Source: three-view drawing plus pictorial views. Frame: mm from the lowest corner of the part. Give positions to 0.01 mm unless a question says otherwise; leave off trailing zeros. Write each loop counter-clockwise with the first axis right and the second up, starting at its lowest first coordinate (ties: lowest second). Pieces come first, ordered by that corner, then holes. Notation, with made-up numbers: M -33.5,-4.75 L -21.5,-4.75 A25 ccw -21.5,9.25 Z; hole C 46.5,76 d5. An arc over 180 degrees is marked long. Return JSON: item names as keys, results as strings.
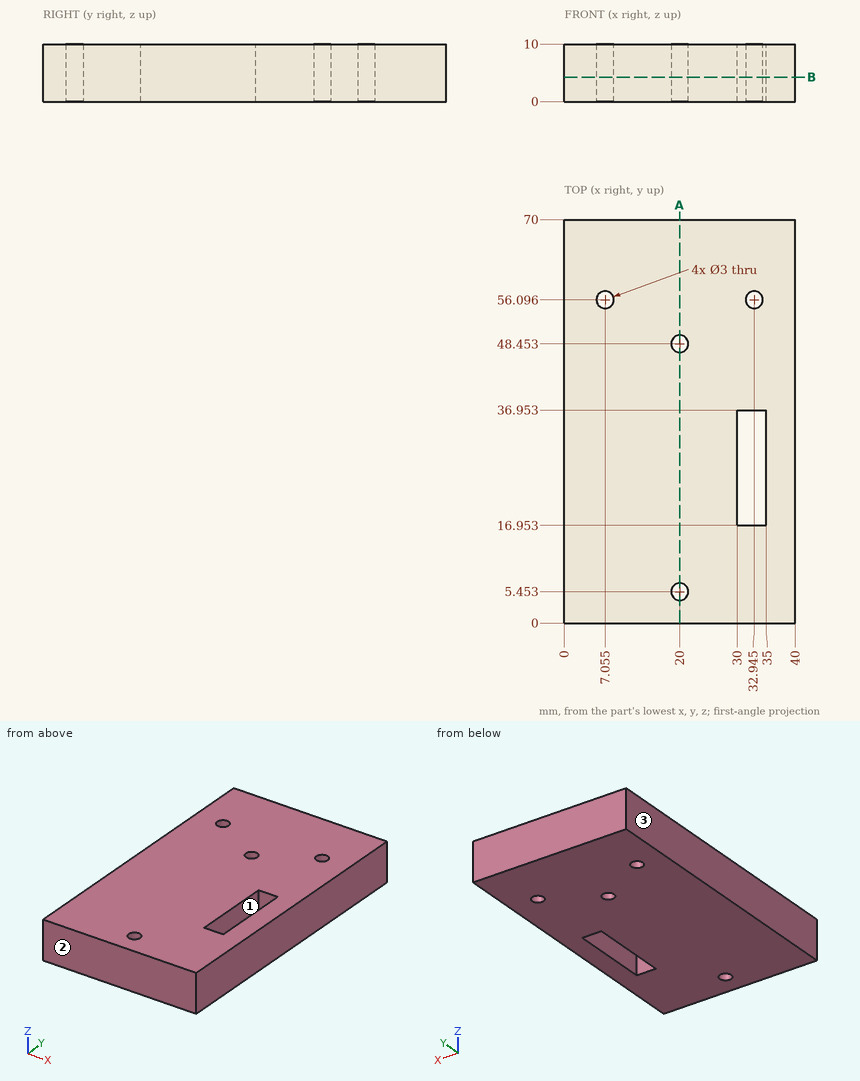
1) Line query: line 1 (Y direction, x = 20, z = 5); line 2 (X direction, y = 30, z = 7); line 3 (Y direction, x = 7, z = 6.5) (1 decimal). Output: solid intervals per line, ascending. Write a range as [from, to].
Numbers:
{"line 1": "y = [0, 3.95], [6.95, 46.95], [49.95, 70]", "line 2": "x = [0, 30], [35, 40]", "line 3": "y = [0, 54.6], [57.6, 70]"}
2) Draft query along X for the marked faces 1, 2 and 3. Return one class per face: released by +X, released by -X, zero draft, split by the parting line, or undercut.
Numbers:
{"face 1": "undercut", "face 2": "zero draft", "face 3": "released by -X"}
3) Cut plane A-A, the plane x = 20. Return the cut outline in (y, z), then the cut area to 3 significant figures.
Numbers:
{"outline": "M 0,0 L 3.95,0 L 3.95,10 L 0,10 Z; M 6.95,0 L 46.95,0 L 46.95,10 L 6.95,10 Z; M 49.95,0 L 70,0 L 70,10 L 49.95,10 Z", "area": "640 mm²"}
4) Contact query for a flat-ended pin moving along its axis: pin 1 Ø2.5 at (x, y) = (20, 48.45) entering from +Z. Output: stop coordinate, or through.
Numbers:
{"pin 1": "passes through"}
5) Cut plane B-B, the plane z = 4.25. Return the cut outline in (x, y) (1 decimal).
Numbers:
{"outline": "M 0,0 L 40,0 L 40,70 L 0,70 Z; hole C 7.1,56.1 d3; hole C 20,5.5 d3; hole C 20,48.5 d3; hole M 30,17 L 35,17 L 35,37 L 30,37 Z; hole C 32.9,56.1 d3"}
